from build123d import *

# Parameters (mm, degrees)
F1_DEPTH = 10.25
F3_DEPTH = 2.25


with BuildPart() as f1:
    # F0 (on Top) → F1 (new body)
    with BuildSketch(Plane.XY):
        with BuildLine():
            Line((-16, -19), (16, -19))
            ThreePointArc((16, -19), (21.656854, -16.656854), (24, -11))
            Line((24, -11), (24, 11))
            ThreePointArc((24, 11), (21.656854, 16.656854), (16, 19))
            Line((16, 19), (-16, 19))
            ThreePointArc((-16, 19), (-21.656854, 16.656854), (-24, 11))
            Line((-24, 11), (-24, -11))
            ThreePointArc((-24, -11), (-21.656854, -16.656854), (-16, -19))
        make_face()
    extrude(amount=F1_DEPTH)

    # F2 (on face) → F3 (join)
    with BuildSketch(Plane.XY.offset(10.25)):
        with BuildLine():
            Line((9, 21.85), (-16, 21.85))
            ThreePointArc((-16, 21.85), (-21.656854, 19.506854), (-24, 13.85))
            Line((-24, 13.85), (-24, 11))
            ThreePointArc((-24, 11), (-21.656854, 16.656854), (-16, 19))
            Line((-16, 19), (10, 19))
            Line((10, 19), (10, 20.85))
            ThreePointArc((10, 20.85), (9.707107, 21.557107), (9, 21.85))
        make_face()
        with BuildLine():
            ThreePointArc((-16, -19), (-21.656854, -16.656854), (-24, -11))
            Line((-24, -11), (-24, -13.85))
            ThreePointArc((-24, -13.85), (-21.656854, -19.506854), (-16, -21.85))
            Line((-16, -21.85), (9, -21.85))
            ThreePointArc((9, -21.85), (9.707107, -21.557107), (10, -20.85))
            Line((10, -20.85), (10, -19))
            Line((10, -19), (-16, -19))
        make_face()
        with BuildLine():
            ThreePointArc((-16, 19), (-21.656854, 16.656854), (-24, 11))
            Line((-24, 11), (-24, -11))
            ThreePointArc((-24, -11), (-21.656854, -16.656854), (-16, -19))
            Line((-16, -19), (10, -19))
            Line((10, -19), (10, 19))
            Line((10, 19), (-16, 19))
        make_face()
    extrude(amount=-F3_DEPTH)


solid = f1.part
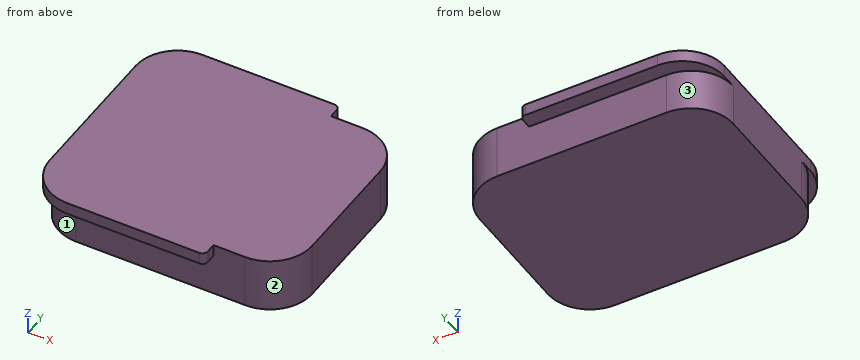
Check sheet for the modelled part. Datum: model origin and axes. Units: mm. Face numbers are marked on the shaded views. A direction names the side the tool comes from. Round coordinates to 2 decimals unless told otherwise and drop trailing zeros. Loops run counter-clockwise (first coordinate to the right, second up) from the corner with the lowest first, then second, coordinate; pieces in that order, holes last.
1. Sectioned sample at A-A on x = 4. Record the boundary of the cut face in (y, z).
2. Scan lines: probe 1 along Y at (x, z) = (-15, 4.5); probe 2 along X at (y, z) = (16, 8.75) (3 decimals); probe 3 along Y at (x, z) = (-22, 4.25). Record each from-to range of solid material in increasing order.
3. Sectioned sample at B-B on z = 4.75. Record the boundary of the cut face in (x, y).
4. Gauge pin test, flat ends, axial feed: pin 1 Ø12 at (x, y) = (-8.5, 15.5) entering from -Z; pin 2 Ø2 at (x, z) = (-17.5, 2) entering from -Y; pin 3 Ø6 at (y, z) = (-14.5, 8) entering from +X. Record the tip position at first contact, or that the pin passes through.
5. Set-up check for the marked faces 1, 2 and 3: record each of +Z, -Z, +X, -X, +Y, -Y from which the full face is reachable in a straight line by a thin tool's end or side.
6. Sectioned sample at C-C on x = 17.5. Record the boundary of the cut face in (y, z), and give its area (3 significant figures).
Recorded:
1. outline: (-21.85, 8) - (-19, 8) - (-19, 0) - (19, 0) - (19, 8) - (21.85, 8) - (21.85, 10.25) - (-21.85, 10.25) - close
2. probe 1: y = -19 to 19
2. probe 2: x = -23.706 to 22.245
2. probe 3: y = -16.29 to 16.29
3. outline: (-24, -11) arc R8 ccw to (-16, -19) - (16, -19) arc R8 ccw to (24, -11) - (24, 11) arc R8 ccw to (16, 19) - (-16, 19) arc R8 ccw to (-24, 11) - close
4. pin 1: stops at z = 0
4. pin 2: stops at y = -18.98
4. pin 3: stops at x = 23.98
5. face 1: -Z, -X, -Y
5. face 2: +Z, -Z, +X, -Y
5. face 3: -Z, -X, +Y
6. outline: (-18.86, 0) - (18.86, 0) - (18.86, 10.25) - (-18.86, 10.25) - close
6. area: 387 mm2
